Can you work these out from the drawing? Everything is in mm from the part's minimum corner. Coordinates: 2 decimals unless noted, no trailing zeros. Loops run counter-clockwise (first coordinate to the right, second up) from the corner with the lowest first, then second, coordinate; pieces in that order, holes last. Notation, with made-up numbers: M 13,9 L 20,9 A18 cw 20,14 Z; hole C -13.75,52 d9. An arc over 180 degrees is marked long. Use CSV: the item, a comma, the result in double quotes. Start each with the question number.
Q1. Please list where these lines run through material, in increasing order: probe 1 along Y at (x, z) = (9, 3.3); probe 2 along X at (y, z) = (10, 2.6); probe 3 along X at (y, z) = (16.5, 49). Write a range as [from, to].
Q2. For pin 1 Ø3 at (x, y) = (8, 3) entering from -Z; pin 2 Ø1.6 at (x, y) = (9, 10) entering from -Z, each with a flat end and sliding along its axis, tell me the tip position at first contact or that it passes through.
Q3. If we section it at A-A (z = 15): Please give me the cut outline in (x, y).
Q4. If we section it at B-B (x = 2.25): Please give me the cut outline in (y, z).
Q5. If we section it at C-C (x = 16.75): Please give me the cut outline in (y, z), and give its area (3 significant figures).
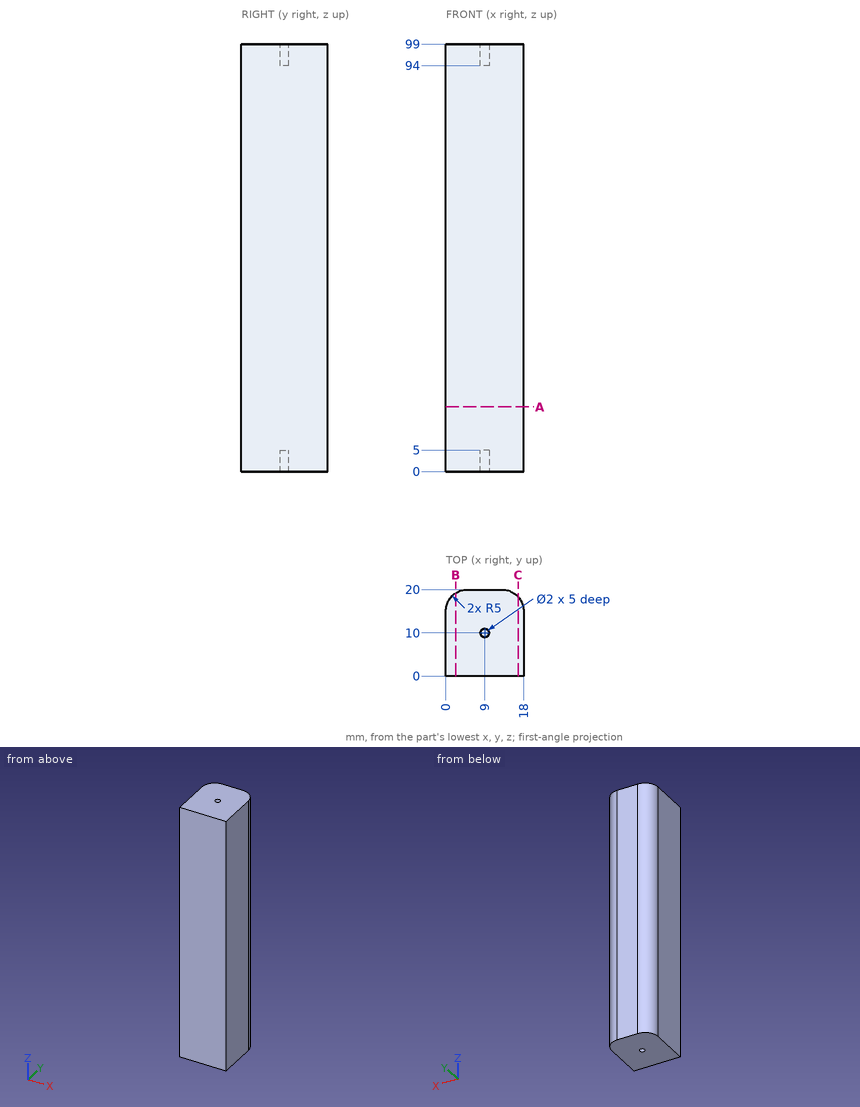
Results below:
1,probe 1,"[0, 9], [11, 20]"
1,probe 2,"[0, 8], [10, 18]"
1,probe 3,"[0.23, 17.77]"
2,pin 1,"z = 0"
2,pin 2,"z = 5"
3,outline,"M 0,0 L 18,0 L 18,15 A5 ccw 13,20 L 5,20 A5 ccw 0,15 Z"
4,outline,"M 0,0 L 19.18,0 L 19.18,99 L 0,99 Z"
5,outline,"M 0,0 L 18.31,0 L 18.31,99 L 0,99 Z"
5,area,"1,810 mm^2"
